The model under review builds one solid part; all positions refer to its coordinate system, in mm. A direction names the side the tool comes from. Round coordinates to 2 decimals unless told otherwise and drop trailing zeros. Order: outer loops, then holes, each group sorted by start corner. A loop starts at its lowest first (then second) coordinate and runs counter-clockwise, first axis right, second up. Notation, with made-up numbers: M 7.25,-30 L 54.25,-30 A10 ccw 54.25,-18 Z; hole C -1,55.25 d7. An arc over 180 degrees is marked long. Use a Markdown table: item, result. Add a question column.
1. For faces 1 (the cylindrical face through (0.33, -35, 152.48)), 2 (the flat face through (0, -59.75, 150)), list the 3-axis set-ups (+Z, -Z, +X, -X, +Y, -Y) from which the entire face can be reached by the end or side of a thin tool; tool diameter is ignored.
2. Consider section D-D on x = -5. State the section outline as (y, z) points.
3. Consider section B-B on z = 150. State the section outline as (x, y) points, then the cut area to 3 significant figures.
4. To check wall thickness, follow probe 1 along Y at (x, z) = (-0.5, 146.5); probe 2 along X at (y, z) = (-21.5, 152.25); probe 3 along Z at (x, y) = (-4.75, -57). State the ranges of each line that lie inside material, in increasing order.
5. Insertion check: P1, Ø8, axis at x = 1.5, y = -27, coming from the +Z side; P2, Ø6, axis at x = -2, y = -29, coming from the -Z side; P3, Ø4, axis at x = -4, y = -47, coming from the +Z side. Each pin has a flat end and moves straight along its axis. Give the tip position at first contact, or say it passes through.
6. Consider section C-C on y = -42.5. State the section outline as (x, z) points, then the cut area to 3 significant figures.
7. Consider section A-A on x = 0. State the section outline as (y, z) points, then the cut area to 3 significant figures.
from build123d import *

# Parameters (mm, degrees)
SKETCH143_R             = 2.5
PAD073_DEPTH            = 42
SKETCH142_W             = 15
SKETCH142_H             = 15
PAD074_DEPTH            = 7
FILLET002_R             = 3
BODY042_PLACEMENT_ANGLE = 180


with BuildPart() as part:
    # Sketch143 → Pad073 (new body)
    with BuildSketch(Plane.XZ):
        Circle(SKETCH143_R)
    extrude(amount=-PAD073_DEPTH)

    # Sketch142 (on Face3 of Pad073) → Pad074 (join)
    with BuildSketch(Plane(origin=(0, 42, 0), x_dir=(1, 0, 0), z_dir=(0, 1, 0))):
        Rectangle(SKETCH142_W, SKETCH142_H)
    extrude(amount=-PAD074_DEPTH)

    # Fillet002
    fillet002_edges = [part.edges().sort_by_distance(p)[0] for p in [
        (7.5, 38.5, -7.5),
        (7.5, 38.5, 7.5),
        (-7.5, 38.5, 7.5),
        (-7.5, 38.5, -7.5),
    ]]
    fillet(fillet002_edges, radius=FILLET002_R)


with BuildPart() as part_1:
    # Body042 placement: moved
    add(part.part.moved(Location((0, -17.75, 150))).rotate(Axis((0, -17.75, 150), (0, 0, 1)), BODY042_PLACEMENT_ANGLE))


solid = part_1.part
Answer block:
| question | item | result |
|---|---|---|
| 1 | face 1 | +Y |
| 1 | face 2 | +Z, -Z, +X, -X, -Y |
| 2 | outline | M -59.75,142.54 L -52.75,142.54 L -52.75,157.46 L -59.75,157.46 Z |
| 3 | outline | M -7.5,-59.75 L 7.5,-59.75 L 7.5,-52.75 L 2.5,-52.75 L 2.5,-17.75 L -2.5,-17.75 L -2.5,-52.75 L -7.5,-52.75 Z |
| 3 | area | 280 mm^2 |
| 4 | probe 1 | -59.75 to -52.75 |
| 4 | probe 2 | -1.09 to 1.09 |
| 4 | probe 3 | 142.51 to 157.49 |
| 5 | P1 | z = 152.5 |
| 5 | P2 | z = 147.5 |
| 5 | P3 | z = 151.5 |
| 6 | outline | C 0,150 d5 |
| 6 | area | 19.6 mm^2 |
| 7 | outline | M -59.75,142.5 L -52.75,142.5 L -52.75,147.5 L -17.75,147.5 L -17.75,152.5 L -52.75,152.5 L -52.75,157.5 L -59.75,157.5 Z |
| 7 | area | 280 mm^2 |
